The model under review builds one solid part; all positions refer to its coordinate system, in mm. Coordinates: 2 decimals unless noted, no trailing zeros. Order: outer loops, then holes, each group sorted by start corner. A loop starts at its lowest first (then second) coordinate and runs counter-clockwise, first axis right, second up. Notation, with made-up numbers: (21, -16) -> (29, -16) arc R32 cw to (29, 18) -> close; hole circle Ø1 at (-6.5, -36.5). An arc over 180 degrees is marked (long way). Use one line per item in the form item = value.
from build123d import *

# Parameters (mm, degrees)
BOSS_EXTRUDE1_DEPTH = 2
SKETCH3_R           = 0.0635


with BuildPart() as part:
    # Sketch1 → Boss-Extrude1 (new body)
    with BuildSketch(Plane(origin=(0, 0, 0), x_dir=(1, 0, 0), z_dir=(0, 1, 0))):
        with BuildLine():
            Line((-2.075, 1.75), (2.075, 1.75))
            ThreePointArc((2.075, 1.75), (2.714429038, 0), (2.075, -1.75))
            Line((2.075, -1.75), (-2.075, -1.75))
            ThreePointArc((-2.075, -1.75), (-2.714429038, 0), (-2.075, 1.75))
        make_face()
    extrude(amount=BOSS_EXTRUDE1_DEPTH)

    # Sweep1: sweep along a path in Sketch2
    with BuildLine(Plane.XY) as sweep1_path:
        Line((-2.075, 0), (-2.286, -26))
    # Sketch3 → Sweep1 (sweep)
    with BuildSketch(Plane.XZ):
        with Locations((-1.27, 0)):
            Circle(SKETCH3_R)
    sweep1 = sweep(path=sweep1_path.line)

    # Mirror1: Sweep1 across plane
    add(sweep1.mirror(Plane(origin=(0, 0, 0), x_dir=(0, 0, 1), z_dir=(1, 0, 0))))


solid = part.part
Item 1: To check wall thickness, follow L1, parallel to Y at x = -0.1, z = -1.25; L2, parallel to X at y = 0.25, z = 0.1. State the ranges of each line that lie inside material, in increasing order. Write a range as from..to.
Results found:
L1 = 0..2
L2 = -2.71..2.71
Item 2: We need section B-B (z = 0.8). Write out the cut boundary in (x, y).
Results found:
outline = (-2.59, 0) -> (2.59, 0) -> (2.59, 2) -> (-2.59, 2) -> close
Item 3: Clearance check with a flat-ended pin moving along its axis: pin 1 (3 mm diameter, centred on x = -2, y = -11.5, fed in from -Z). State where the tip first meets the part, or that it passes through.
Results found:
pin_1 = -0.06
Item 4: We need section A-A (x = 0.5). Write out the cut boundary in (y, z), plus the area to 3 significant figures.
Results found:
outline = (0, -1.75) -> (2, -1.75) -> (2, 1.75) -> (0, 1.75) -> close
area = 7.00 mm²
